Answer from the drawing. Dimensions are ordinates in mm from the lowest x, y and z of the part. A direction names the side the tool comes from. Give positions to 0.01 mm unless a question says otherwise; leave off trailing zeros. Loops run counter-clockwise (first coordinate to the right, second up) from the corner with the lowest first, then second, coordinate; pieces in that order, holes last. Notation, with made-up numbers: (58.25, 61) - (73.25, 61) arc R15 cw to (73.25, 66) - close; hole circle Ø7 at (-36.5, 44.25). An arc over 180 degrees is marked (long way). One line per item, written item: value.
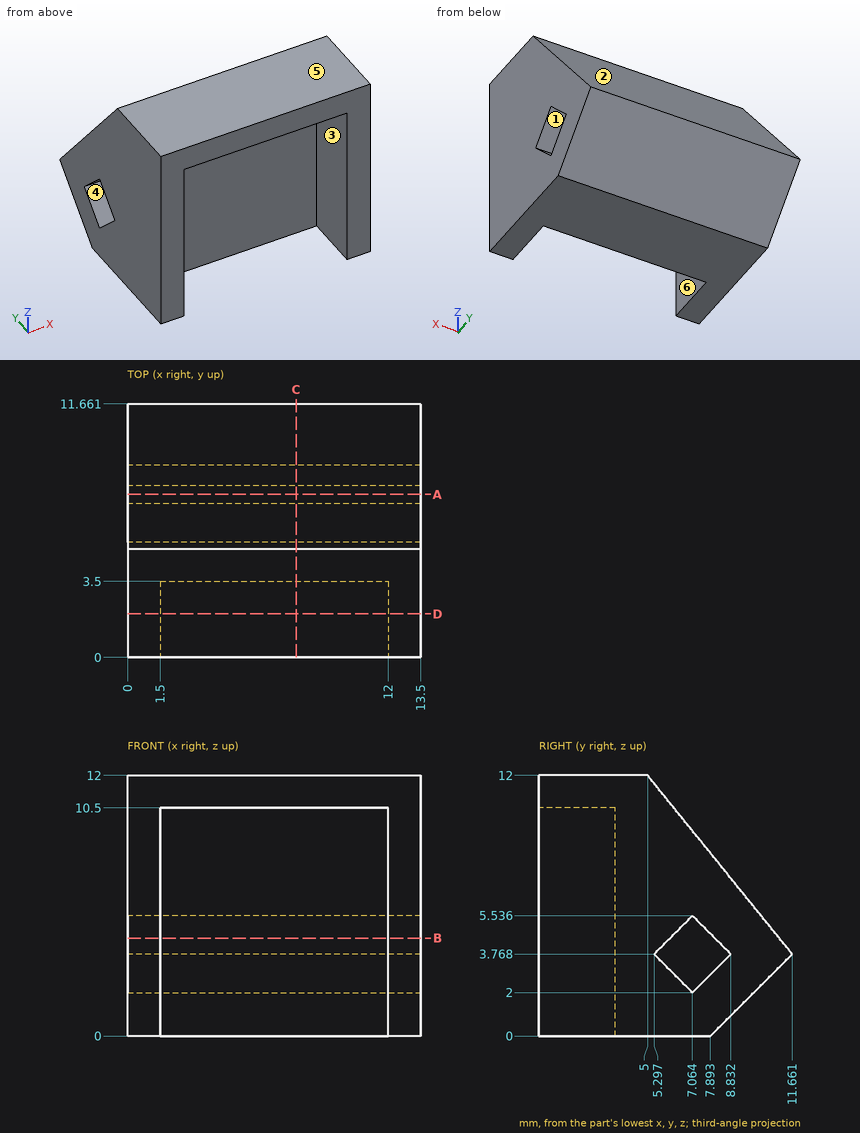
1. The mould has two halves that part along Z. Classify the marked faces 4, 5 and 6: released by +Z, released by -Z, zero draft, split by the parting line, or undercut.
Output:
face 4: undercut
face 5: released by +Z
face 6: zero draft
2. Section C-C (x = 7.75) is taken. Write down the section's boundary in (y, z) (1 decimal).
Output:
outline: (0, 10.5) - (3.5, 10.5) - (3.5, 0) - (7.9, 0) - (11.7, 3.8) - (5, 12) - (0, 12) - close; hole (5.3, 3.8) - (7.1, 2) - (8.8, 3.8) - (7.1, 5.5) - close
3. Flat-ended cylindrical pins translate along their axes: pin 1 Ø3 at (x, z) = (2.5, 4) entering from +Y; pin 2 Ø1 at (x, y) = (5.5, 2) entering from -Z; pin 3 Ø3 at (x, z) = (9, 5) entering from -Y. Find the tip coordinate at first contact, or state that the pin passes through.
Output:
pin 1: stops at y = 11.66
pin 2: stops at z = 10.5
pin 3: stops at y = 3.5
4. Section A-A (y = 7.5) is taken. Write down the section's boundary in (x, z) (1 decimal).
Output:
outline: (0, 0) - (13.5, 0) - (13.5, 2.4) - (0, 2.4) - close; (0, 5.1) - (13.5, 5.1) - (13.5, 8.9) - (0, 8.9) - close
5. For the marked faces 1, 2 and 3, determine the directions among +Z, -Z, +X, -X, +Y, -Y from which every point of the face is accessible in a straight line to the end or side of a thin tool.
Output:
face 1: +X, -X
face 2: +Z, +X, -X, +Y
face 3: -Z, -Y
6. Section D-D (y = 2) is taken. Write down the section's boundary in (x, z).
Output:
outline: (0, 0) - (1.5, 0) - (1.5, 10.5) - (12, 10.5) - (12, 0) - (13.5, 0) - (13.5, 12) - (0, 12) - close
7. Section B-B (z = 4.5) is taken. Write down the section's boundary in (x, y).
Output:
outline: (0, 0) - (1.5, 0) - (1.5, 3.5) - (12, 3.5) - (12, 0) - (13.5, 0) - (13.5, 6.03) - (0, 6.03) - close; (0, 8.1) - (13.5, 8.1) - (13.5, 11.07) - (0, 11.07) - close
8. Find the intervals of material crossed by line 1 along X through (y, z) = (1, 8.25); line 2 along Z through (x, y) = (8.25, 1.5); line 3 along Y through (x, z) = (2.5, 3) (1 decimal), in increasing order.
Output:
line 1: x = 0 to 1.5, 12 to 13.5
line 2: z = 10.5 to 12
line 3: y = 3.5 to 6.1, 8.1 to 10.9
